```python
from build123d import *

# Parameters (mm, degrees)
F1_DEPTH = 50.8
F3_DEPTH = 12.7
F4_R     = 5.569694
F5_DEPTH = 50.8


with BuildPart() as f1:
    # F0 (on Front) → F1 (new body)
    with BuildSketch(Plane.XZ):
        Polygon((-46.874546, 0), (0, 0), (-25.861818, 40.293638), (-46.874546, 40.293638), align=None)
    extrude(amount=F1_DEPTH)

    # F2 (on Front) → F3 (join)
    with BuildSketch(Plane.XZ):
        Polygon((-47.105454, 47.220912), (-47.105454, 0), (10.852728, 0), (-21.705456, 47.220912), align=None)
    extrude(amount=F3_DEPTH)

    # F4 (on face) → F5 (cut)
    with BuildSketch(Plane(origin=(-46.874546, 0, 0), x_dir=(0, -1, 0), z_dir=(-1, 0, 0))):
        with Locations((31.75, 20.146819)):
            Circle(F4_R)
    extrude(amount=-F5_DEPTH, mode=Mode.SUBTRACT)


solid = f1.part
```
Part model, mm, in its own coordinate system. A direction names the side the tool comes from. Round coordinates to 2 decimals unless told otherwise and drop trailing zeros. Order: outer loops, then holes, each group sorted by start corner. A loop starts at its lowest first (then second) coordinate and runs counter-clockwise, first axis right, second up. Notation, with made-up numbers: M 55.5,-30 L 67.5,-30 A5 ccw 67.5,-21 Z; hole C -22.75,19.5 d11. An arc over 180 degrees is marked long. Put each result on its own line as item: value. Start each with the question number.
1. Slice it at A-A on y = -31.75. List the corners of the cut face in (x, z), then the cut area to 3 significant figures.
2. Slice it at B-B on z = 16.5. List the corners of the cut face in (x, y), then the cut area to 3 significant figures.
3. Tool access for faces 1 (the face through (-15.62, -27.25, 24.34)), 2 (the face through (-46.875, -27, 25)), 3 (the face through (-36, -31, 40.294)): list every direction of +Z, -Z, +X, -X, +Y, -Y with a clear straight run to the whole face (end or side of a thin tool).
4. Slice it at D-D on z = 6.5. List the corners of the cut face in (x, y), then the cut area to 3 significant figures.
5. Slice it at C-C on x = -34. List the corners of the cut face in (y, z), then the cut area to 3 significant figures.
6. Two-plate mould, pull along Z, no slides. Class faces 4 (the face through (-28.34, -30.54, 14.71)), 5 (the face through (-16, -12.7, 29)), 6 (the face through (-34, -6, 47.221)): +Z half, -Z half, draft (parallel to the pull), parting line (faces both ways), or undercut.
7. Drill centre lines: probe 1 along Z at (x, y) = (-38, -31.75); probe 2 along Z at (x, y) = (-41.5, -48); probe 3 along Z at (x, y) = (-22, -31.75). Where is each one in solid material? Low to high. Write a range as [from, to].
8. Drop flat-ended pins along their axis: pin 1 (23 mm diameter, centred on x = -34, y = -39, fed in from +Z); pin 2 (14 mm diameter, centred on x = -4, z = 30, fed in from -Y); pin 3 (19 mm diameter, centred on y = -25.5, z = 18, fed in from -X). Give the stop position or say it passes through.
Findings:
1. outline: M -46.87,0 L 0,0 L -9.36,14.58 L -46.87,14.58 Z; M -46.87,25.72 L -16.51,25.72 L -25.86,40.29 L -46.87,40.29 Z
1. area: 990 mm2
2. outline: M -47.11,-12.7 L -46.87,-12.7 L -46.87,-27.54 L -10.59,-27.54 L -10.59,-12.7 L -0.52,-12.7 L -0.52,0 L -47.11,0 Z; M -46.87,-50.8 L -10.59,-50.8 L -10.59,-35.96 L -46.87,-35.96 Z
2. area: 1,670 mm2
3. face 1: +Z, +X, -Y
3. face 2: +Z, -Z, -X, -Y
3. face 3: +Z, +X, -X, -Y
4. outline: M -47.11,-12.7 L -46.87,-12.7 L -46.87,-50.8 L -4.17,-50.8 L -4.17,-12.7 L 6.37,-12.7 L 6.37,0 L -47.11,0 Z
4. area: 2,310 mm2
5. outline: M -50.8,0 L 0,0 L 0,47.22 L -12.7,47.22 L -12.7,40.29 L -50.8,40.29 Z; hole C -31.75,20.15 d11.14
5. area: 2,040 mm2
6. face 4: undercut
6. face 5: draft
6. face 6: +Z half
7. probe 1: [0, 14.58], [25.72, 40.29]
7. probe 2: [0, 40.29]
7. probe 3: [0, 14.58], [25.72, 34.28]
8. pin 1: z = 40.29
8. pin 2: y = -12.7
8. pin 3: x = -46.87
